Verification items for the finished model (mm, model axes). Face numbers are marked on the shaded views. A direction names the side the tool comes from. Give positions to 0.01 mm unless a question says otherwise; leave off trailing zeros. Write each loop counter-clockwise with the first axis right and the second up, starting at its lowest first coordinate (ties: lowest second). Pieces come first, ordered by that corner, then holes. Notation, with made-up numbers: (-23, 14.25) -> (-11, 14.25) arc R17 cw to (-11, 40.25) -> close; hole circle Ø6 at (52, 62.25). An arc over 180 degrees is marked (long way). Write item = value, one per line.
from build123d import *

# Parameters (mm, degrees)
SKETCH1_W           = 150
SKETCH1_H           = 100
BOSS_EXTRUDE1_DEPTH = 5
SKETCH2_W           = 150
SKETCH2_H           = 31.506784204
BOSS_EXTRUDE2_DEPTH = 5
SKETCH4_W           = 31.506784204
SKETCH4_H           = 105
BOSS_EXTRUDE3_DEPTH = 5
SKETCH5_W           = 155
SKETCH5_H           = 31.506784204
BOSS_EXTRUDE4_DEPTH = 5
SKETCH6_W           = 31.506784204
SKETCH6_H           = 110
BOSS_EXTRUDE5_DEPTH = 5


with BuildPart() as part:
    # Sketch1 → Boss-Extrude1 (new body)
    with BuildSketch(Plane.XY):
        Rectangle(SKETCH1_W, SKETCH1_H)
    extrude(amount=BOSS_EXTRUDE1_DEPTH)

    # Sketch2 → Boss-Extrude2 (add)
    with BuildSketch(Plane.XZ.offset(50)):
        with Locations((0, 15.753392102)):
            Rectangle(SKETCH2_W, SKETCH2_H)
    extrude(amount=BOSS_EXTRUDE2_DEPTH)

    # Sketch4 → Boss-Extrude3 (add)
    with BuildSketch(Plane(origin=(75, 0, 0), x_dir=(0, 0, -1), z_dir=(1, 0, 0))):
        with Locations((-15.753392102, -2.5)):
            Rectangle(SKETCH4_W, SKETCH4_H)
    extrude(amount=BOSS_EXTRUDE3_DEPTH)

    # Sketch5 → Boss-Extrude4 (add)
    with BuildSketch(Plane(origin=(0, 50, 0), x_dir=(1, 0, 0), z_dir=(0, 1, 0))):
        with Locations((2.5, -15.753392102)):
            Rectangle(SKETCH5_W, SKETCH5_H)
    extrude(amount=BOSS_EXTRUDE4_DEPTH)

    # Sketch6 → Boss-Extrude5 (add)
    with BuildSketch(Plane.ZY.offset(75)):
        with Locations((15.753392102, 0)):
            Rectangle(SKETCH6_W, SKETCH6_H)
    extrude(amount=BOSS_EXTRUDE5_DEPTH)


solid = part.part
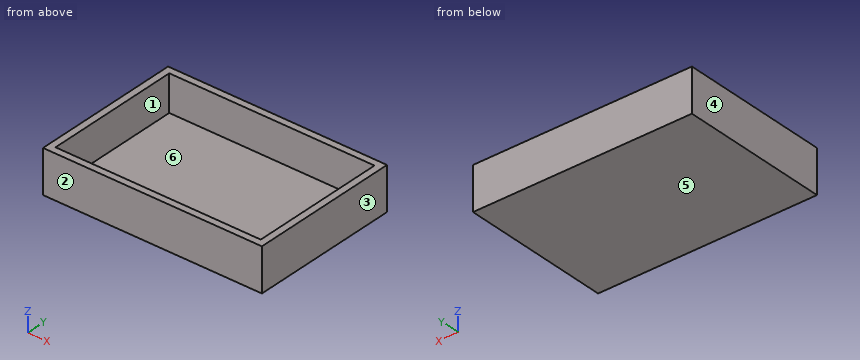
Item 1: Mould release check, pull along X, two halves, no side actions. Record for the marked faces 3, 4, 5 and 6: +X half, -X half, draft (parallel to the pull), parting line (faces both ways), or undercut.
Response values:
face_3 = +X half
face_4 = -X half
face_5 = draft
face_6 = undercut
Item 2: Sectioned sample at B-B on z = 14.5. Record the cut outline in (x, y).
Response values:
outline = (-80, -55) -> (80, -55) -> (80, 55) -> (-80, 55) -> close; hole (-75, -50) -> (75, -50) -> (75, 50) -> (-75, 50) -> close
Item 3: Go/stop test with a flat-tipped pin: P1, Ø1, axis at x = -4.5, y = -41, coming from the +Z side. Record where the tip stops, or that it passes through.
Response values:
P1 = 5
Item 4: Sectioned sample at A-A on y = 9. Record the cut outline in (x, z), then the cut area to 3 significant figures.
Response values:
outline = (-80, 0) -> (80, 0) -> (80, 31.51) -> (75, 31.51) -> (75, 5) -> (-75, 5) -> (-75, 31.51) -> (-80, 31.51) -> close
area = 1,070 mm^2
Item 5: Sectioned sample at C-C on x = -24.5. Record the cut outline in (y, z).
Response values:
outline = (-55, 0) -> (55, 0) -> (55, 31.51) -> (50, 31.51) -> (50, 5) -> (-50, 5) -> (-50, 31.51) -> (-55, 31.51) -> close
Item 6: Material ranges on line 1 (X direction, y = -24, z = 22.5); line 2 (Y direction, x = -22, z = 10.5); line 3 (Z direction, x = -27.5, y = 39), recorded low to high.
Response values:
line_1 = -80 to -75, 75 to 80
line_2 = -55 to -50, 50 to 55
line_3 = 0 to 5
Item 7: Set-up check for the marked faces 1 and 2: record each of +Z, -Z, +X, -X, +Y, -Y from which the full face is reachable in a straight line by a thin tool's end or side.
Response values:
face_1 = +Z
face_2 = +Z, -Z, +X, -X, -Y
